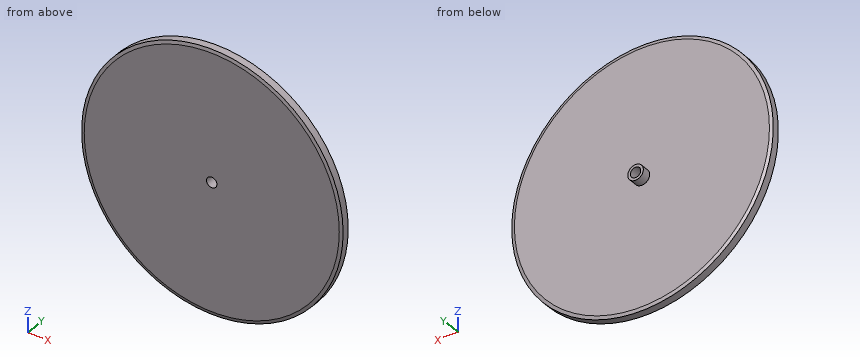
from build123d import *

# Parameters (mm, degrees)
CHAMFER_1_SIZE           = 1.25
CHAMFER_1_SIZE2          = 0.334936491
CHAMFER_2_SIZE           = 1.25
CHAMFER_2_SIZE2          = 0.334936491
SKETCH_2_R               = 2
CUT_EXTRUDE_3_DEPTH      = 1
CUT_EXTRUDE_3_DEPTH_BACK = 8


with BuildPart() as part:
    # Эскиз1 → Повернуть2 (revolve)
    with BuildSketch(Plane.XY):
        Polygon((0, 0), (50.5, 0), (50.5, 3.5), (3, 3.5), (3, 7), (0, 7), align=None)
    revolve(axis=Axis((0, 7, 0), (0, -1, 0)))

    # Фаска1
    chamfer_1_edges = [part.edges().sort_by_distance(p)[0] for p in [
        (-50.5, 3.5, 0),
    ]]
    chamfer_1_side = [part.faces().sort_by_distance(p)[0] for p in [
        (-49.071644302, 3.5, 0),
    ]]
    chamfer(chamfer_1_edges, length=CHAMFER_1_SIZE, length2=CHAMFER_1_SIZE2, reference=chamfer_1_side[0])

    # Фаска2
    chamfer_2_edges = [part.edges().sort_by_distance(p)[0] for p in [
        (-50.5, 0, 0),
    ]]
    chamfer_2_side = [part.faces().sort_by_distance(p)[0] for p in [
        (0, 0, 0),
    ]]
    chamfer(chamfer_2_edges, length=CHAMFER_2_SIZE, length2=CHAMFER_2_SIZE2, reference=chamfer_2_side[0])

    # Эскиз2 → Вырез-Вытянуть3 (cut, two sides)
    with BuildSketch(Plane(origin=(0, 0, 0), x_dir=(-1, 0, 0), z_dir=(0, -1, 0))) as cut_extrude_3_sk:
        Circle(SKETCH_2_R)
    extrude(amount=CUT_EXTRUDE_3_DEPTH, mode=Mode.SUBTRACT)
    extrude(cut_extrude_3_sk.sketch, amount=-CUT_EXTRUDE_3_DEPTH_BACK, mode=Mode.SUBTRACT)


solid = part.part
Here's how the part is built. I have some questions about the finished solid (model axes, mm). Coordinates: 2 decimals unless noted, no trailing zeros. Write each loop counter-clockwise with the first axis right and the second up, starting at its lowest first coordinate (ties: lowest second). Pieces come first, ordered by that corner, then holes.
Item 1: Will these pins go through, and if not, where does the flat tip stop? pin 1 (1.5 mm diameter, centred on x = 1, y = 3, fed in from +Z); pin 2 (1.5 mm diameter, centred on x = -2.5, z = 22, fed in from -Y); pin 3 (4 mm diameter, centred on y = 2, z = -21.5, fed in from +X); pin 4 (1 mm diameter, centred on y = 1.5, z = -4, fed in from -X).
Item 2: If I drill on line 1 (Z direction, x = 0, y = 1.75); line 2 (Z direction, x = 0, y = 3.75); line 3 (Y direction, x = 20.5, z = 4), over which ranges is the centre line in solid material (lowest first)?
Item 3: I want a section at B-B on y = 2. Write out the boundary of the cut face in (x, z).
Item 4: I want a section at A-A on x = 0. Write out the boundary of the cut face in (y, z), and give its area (3 significant figures).
Findings below:
1. pin 1: stops at z = 50.5
1. pin 2: stops at y = 0
1. pin 3: stops at x = 46.58
1. pin 4: stops at x = -50.38
2. line 1: z = -50.5 to -2, 2 to 50.5
2. line 2: z = -3 to -2, 2 to 3
2. line 3: y = 0 to 3.5
3. outline: circle Ø101 at (0, 0); hole circle Ø4 at (0, 0)
4. outline: (0, -49.25) - (0.33, -50.5) - (3.17, -50.5) - (3.5, -49.25) - (3.5, -3) - (7, -3) - (7, -2) - (0, -2) - close; (0, 2) - (7, 2) - (7, 3) - (3.5, 3) - (3.5, 49.25) - (3.17, 50.5) - (0.33, 50.5) - (0, 49.25) - close
4. area: 346 mm2
